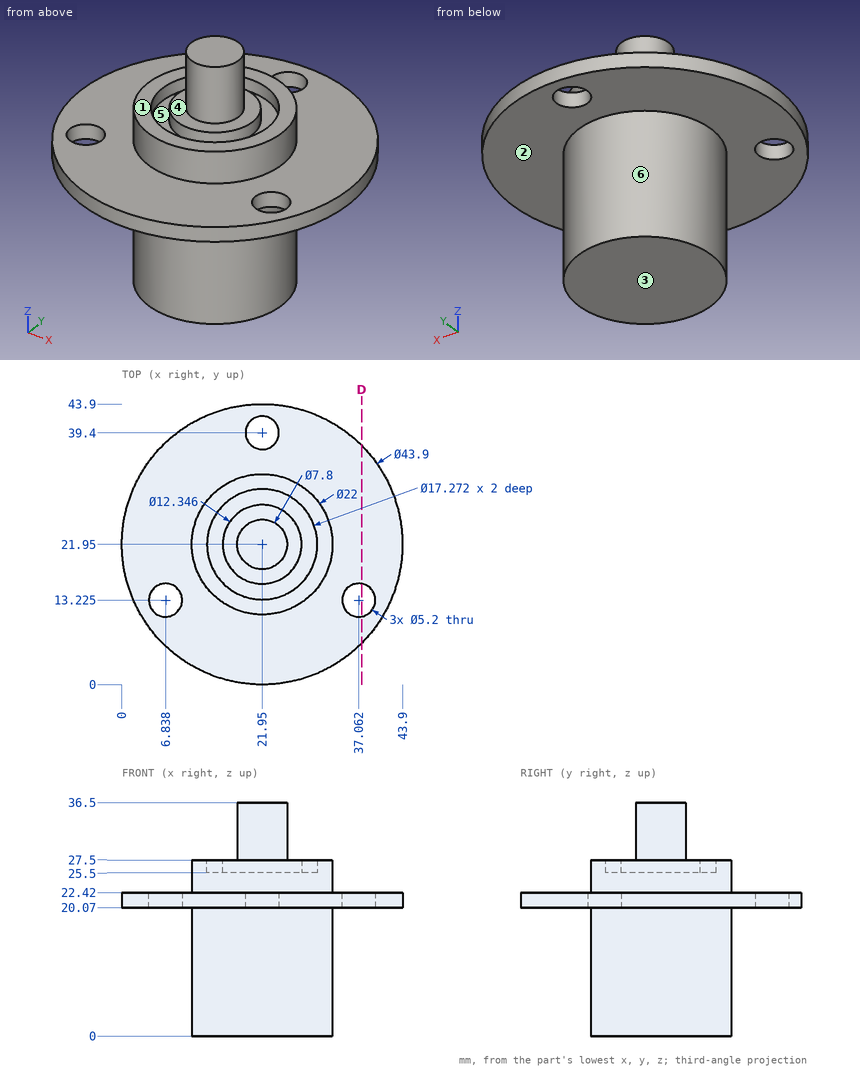
Study the drawing (mm; zero at the part's minimum x, y, z) and answer. A direction names the side the tool comes from. Round coordinates to 2 decimals unless told otherwise and drop trailing zeros. Write each loop counter-clockwise with the first axis right and the second up, starting at its lowest first coordinate (ties: lowest second). Pieces come first, ordered by that corner, then holes. Notation, with made-up numbers: (54, 71.5) - (97, 71.5) arc R7 ccw to (97, 81.5) - close; hole circle Ø11 at (74.25, 19). An arc over 180 degrees is marked (long way). Use a Markdown table: item, result. Add a question column.
1. Consider line 1 (Y direction, x = 21, z = 26); line 2 (Z direction, x = 37.5, y = 25.5); line 3 (Z direction, x = 14, y = 25.5). Determine where each line is inside the solid, lowest interval first.
2. Flat-ended cylindrical pins translate along their axes: P1, Ø3, axis at y = 14.5, z = 20, coming from the -X side; P2, Ø24, axis at x = 19, y = 17, coming from the +Z side; P3, Ø1, axis at x = 26.5, y = 7, coming from the -Z side; P4, Ø10, axis at y = 10.5, z = 10.5, coming from the +X side. Find the tip coordinate at first contact, or state that the pin passes through.
3. The part is cut by section D-D (x = 37.5). Write down the section's boundary in (y, z).
4. A tool of negligible diameter and unlimited length cuts with its end or side. For the marked faces 1, 2 and 3, from which of +Z, -Z, +X, -X, +Y, -Y can it reach the whole face along a straight path? Write none if from no direction.
5. For a pull along Y with two mould halves and no side action, classify the marked faces 4, 5 and 6 as +Y half, -Y half, draft (parallel to the pull), parting line (faces both ways), or undercut.
Reported:
| question | item | result |
|---|---|---|
| 1 | line 1 | 10.99 to 13.37, 15.85 to 28.05, 30.53 to 32.91 |
| 1 | line 2 | 20.07 to 22.42 |
| 1 | line 3 | 0 to 27.5 |
| 2 | P1 | x = 0.82 |
| 2 | P2 | z = 36.5 |
| 2 | P3 | z = 20.07 |
| 2 | P4 | x = 30.86 |
| 3 | outline | (6.46, 20.07) - (10.66, 20.07) - (10.66, 22.42) - (6.46, 22.42) - close; (15.79, 20.07) - (37.44, 20.07) - (37.44, 22.42) - (15.79, 22.42) - close |
| 4 | face 1 | +Z |
| 4 | face 2 | -Z |
| 4 | face 3 | -Z, +X, -X, +Y, -Y |
| 5 | face 4 | draft |
| 5 | face 5 | undercut |
| 5 | face 6 | parting line |
